Drawing for the job (mm, zero at the part's lowest x, y, z). A direction names the side the tool comes from. Coordinates: 2 decimals unless noted, no trailing zeros. Write each loop counter-clockwise with the first axis right and the second up, starting at its lowest first coordinate (ties: lowest second). Pieces come first, ordered by that corner, then holes. Notation, with made-up numbers: (30.25, -25) - (51.25, -25) arc R23 ccw to (51.25, -9) - close; hole circle Ø8 at (-19.5, 64). An arc over 180 degrees is marked (long way). Write each question's results on one line, items separated by ' | '.
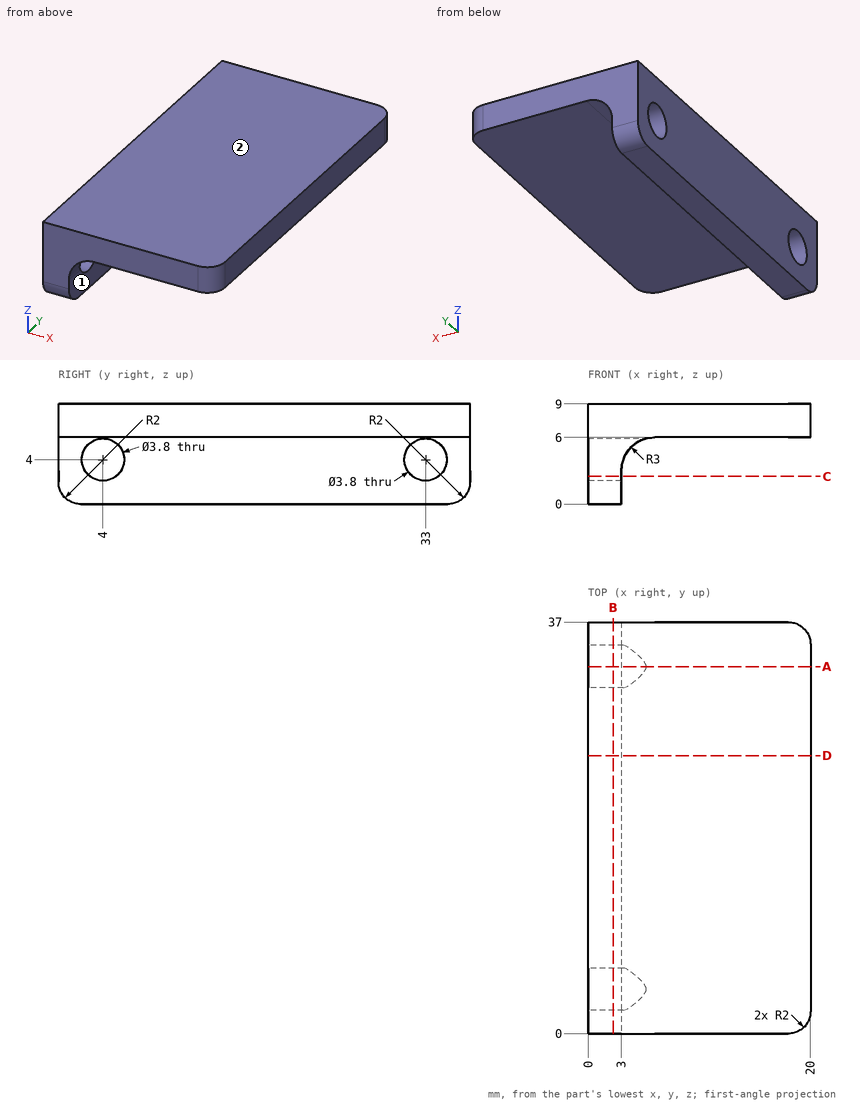
(1) Saw through at C-C on z = 2.5. Write the cut outline in (x, y).
Return value:
outline: (0, 0) - (3, 0) - (3, 2.83) - (0, 2.83) - close; (0, 5.17) - (3, 5.17) - (3, 31.83) - (0, 31.83) - close; (0, 34.17) - (3, 34.17) - (3, 37) - (0, 37) - close
(2) Saw through at B-B on x = 2.25. Write the cut outline in (y, z).
Return value:
outline: (0, 2) arc R2 ccw to (2, 0) - (35, 0) arc R2 ccw to (37, 2) - (37, 9) - (0, 9) - close; hole circle Ø3.8 at (4, 4); hole circle Ø3.8 at (33, 4)
(3) 3-axis set-ups, long thin cutter, end or side, ignore diameter. For the marked faces 1 and 2: which of +Z, -Z, +X, -X, +Y, -Y reach the whole face in a straight line?
Return value:
face 1: -Z, +X, +Y, -Y | face 2: +Z, +X, -X, +Y, -Y
(4) Wall check: line 1 (Y direction, x = 1.5, z = 4); line 2 (Z direction, x = 14.5, y = 2); line 3 (X direction, y = 13.5, z = 1). Give the ranges that are in metal, low to high. Write a range as from..to.
Return value:
line 1: y = 0..2.1, 5.9..31.1, 34.9..37 | line 2: z = 6..9 | line 3: x = 0..3
(5) Saw through at A-A on y = 33. Write the cut outline in (x, z), then the cut area to 3 significant figures.
Return value:
outline: (0, 0) - (3, 0) - (3, 2.1) - (0, 2.1) - close; (0, 5.9) - (5.23, 5.9) arc R3 cw to (6, 6) - (20, 6) - (20, 9) - (0, 9) - close | area: 66.8 mm^2
(6) Saw through at D-D on y = 25. Write the cut outline in (x, z), then the cut area to 3 significant figures.
Return value:
outline: (0, 0) - (3, 0) - (3, 3) arc R3 cw to (6, 6) - (20, 6) - (20, 9) - (0, 9) - close | area: 79.9 mm^2
(7) Flat gauge pins, fed straight in: P1, Ø11, axis at x = 12.5, y = 14.5, coming from the -Z side; P2, Ø1.5, axis at x = 11.5, z = 3.5, coming from the +Y side; P3, Ø3, axis at x = 14.5, z = 5.5, coming from the +Y side; P4, Ø2.5, axis at y = 25, z = 1, coming from the +X side. Where does each tip first touch, or does it go through?
Return value:
P1: stops at z = 6 | P2: passes through | P3: stops at y = 37 | P4: stops at x = 3
